Could you check a few things on this drawing? It's one solid part, dimensions in mm from its lowest x, y, z. Round coordinates to 2 decimals unless told otherwise and drop trailing zeros. Loops run counter-clockwise (first coordinate to the right, second up) from the corner with the lowest first, then second, coordinate; pieces in that order, holes last. Notation, with made-up numbers: M 10.25,61 L 42.25,61 A29 ccw 42.25,93 Z; hole C 11,7.5 d7. An arc over 180 degrees is marked long. Return JSON: item names as keys, results as strings.
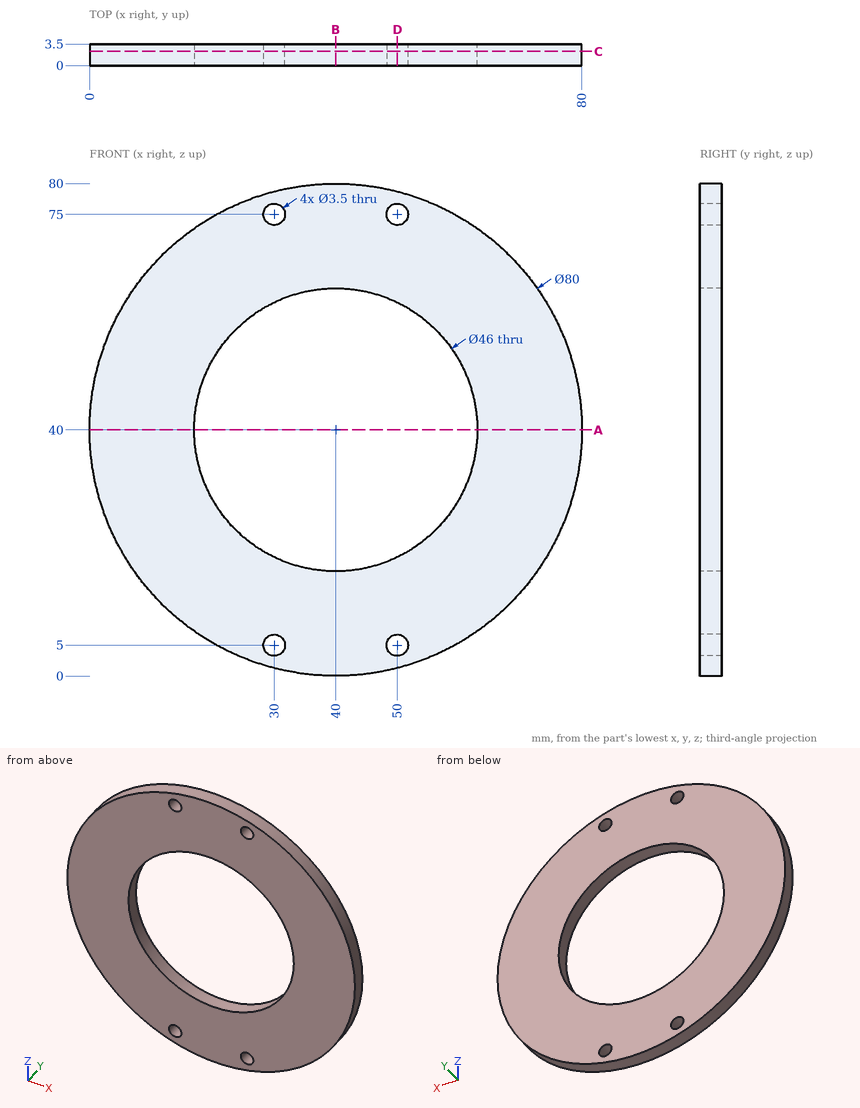
Q1. Suppose I cut it at A-A, the plane z = 40. Please give me the cut outline in (x, y), plus the area to 3 significant figures.
Results:
{"outline": "M 0,0 L 17,0 L 17,3.5 L 0,3.5 Z; M 63,0 L 80,0 L 80,3.5 L 63,3.5 Z", "area": "119 mm2"}
Q2. Suppose I cut it at B-B, the plane x = 40. Please give me the cut outline in (y, z).
Results:
{"outline": "M 0,0 L 3.5,0 L 3.5,17 L 0,17 Z; M 0,63 L 3.5,63 L 3.5,80 L 0,80 Z"}
Q3. I'm going to push flat-ended pins straight in: pin 1 Ø1 at (y, z) = (2, 50.5) entering from +X; pin 2 Ø2 at (x, y) = (50.5, 3) entering from +Z. Where does each tip first touch, or does it pass through?
Results:
{"pin 1": "stops at x = 78.73", "pin 2": "stops at z = 78.86"}
Q4. Suppose I cut it at D-D, the plane x = 50. Please give me the cut outline in (y, z).
Results:
{"outline": "M 0,1.27 L 3.5,1.27 L 3.5,3.25 L 0,3.25 Z; M 0,6.75 L 3.5,6.75 L 3.5,19.29 L 0,19.29 Z; M 0,60.71 L 3.5,60.71 L 3.5,73.25 L 0,73.25 Z; M 0,76.75 L 3.5,76.75 L 3.5,78.73 L 0,78.73 Z"}
Q5. If I drill on line 1 along Z through (x, y) = (50, 0.45); line 2 along Z through (x, y) = (40, 1.6), over which ranges is the centre line in solid material (lowest first)?
Results:
{"line 1": "z = 1.27 to 3.25, 6.75 to 19.29, 60.71 to 73.25, 76.75 to 78.73", "line 2": "z = 0 to 17, 63 to 80"}
Q6. Suppose I cut it at C-C, the plane y = 2.3. Please give me the cut outline in (x, z), plus the area to 3 significant figures.
Results:
{"outline": "C 40,40 d80; hole C 40,40 d46; hole C 30,5 d3.5; hole C 30,75 d3.5; hole C 50,5 d3.5; hole C 50,75 d3.5", "area": "3,330 mm2"}
